```python
from build123d import *

# Parameters (mm, degrees)
EXTRUDE_1_DEPTH     = 20
SKETCH_3_R          = 2.5
CUT_EXTRUDE_1_DEPTH = 4
SKETCH_4_R          = 1.5
CUT_EXTRUDE_2_DEPTH = 14
SKETCH_5_W          = 7.5
SKETCH_5_H          = 8
EXTRUDE_2_DEPTH     = 30
SKETCH_6_R          = 3
CUT_EXTRUDE_3_DEPTH = 6
SKETCH_7_R          = 1.5
CUT_EXTRUDE_4_DEPTH = 6
CHAMFER_1_SIZE      = 2
FILLET_1_R          = 2


with BuildPart() as part:
    # 草图1 → 凸台-拉伸1 (new body)
    with BuildSketch(Plane(origin=(0, 0, 0), x_dir=(1, 0, 0), z_dir=(0, 1, 0))):
        with BuildLine():
            Line((-10.8, 0), (-0.8, 0))
            ThreePointArc((-0.8, 0), (0, 0.8), (0.8, 0))
            Line((0.8, 0), (2.2, 0))
            ThreePointArc((2.2, 0), (3, 0.8), (3.8, 0))
            Line((3.8, 0), (5.2, 0))
            ThreePointArc((5.2, 0), (6, 0.8), (6.8, 0))
            Line((6.8, 0), (8.2, 0))
            ThreePointArc((8.2, 0), (9, 0.8), (9.8, 0))
            Line((9.8, 0), (11.2, 0))
            ThreePointArc((11.2, 0), (12, 0.8), (12.8, 0))
            Line((12.8, 0), (14.2, 0))
            ThreePointArc((14.2, 0), (15, 0.8), (15.8, 0))
            Line((15.8, 0), (17.2, 0))
            ThreePointArc((17.2, 0), (18, 0.8), (18.8, 0))
            Line((18.8, 0), (20.2, 0))
            ThreePointArc((20.2, 0), (21, 0.8), (21.8, 0))
            Line((21.8, 0), (23.2, 0))
            ThreePointArc((23.2, 0), (24, 0.8), (24.8, 0))
            Line((24.8, 0), (26.2, 0))
            ThreePointArc((26.2, 0), (27, 0.8), (27.8, 0))
            Line((27.8, 0), (29.2, 0))
            ThreePointArc((29.2, 0), (30, 0.8), (30.8, 0))
            Line((30.8, 0), (32.2, 0))
            ThreePointArc((32.2, 0), (33, 0.8), (33.8, 0))
            Line((33.8, 0), (35.2, 0))
            ThreePointArc((35.2, 0), (36, 0.8), (36.8, 0))
            Line((36.8, 0), (38.2, 0))
            ThreePointArc((38.2, 0), (39, 0.8), (39.8, 0))
            Line((39.8, 0), (41.2, 0))
            ThreePointArc((41.2, 0), (42, 0.8), (42.8, 0))
            Line((42.8, 0), (44.2, 0))
            ThreePointArc((44.2, 0), (45, 0.8), (45.8, 0))
            Line((45.8, 0), (55.8, 0))
            Line((55.8, 0), (55.8, 8))
            Line((55.8, 8), (-10.8, 8))
            Line((-10.8, 8), (-10.8, 0))
        make_face()
    extrude(amount=EXTRUDE_1_DEPTH)

    # 草图3 → 切除-拉伸1 (cut)
    with BuildSketch(Plane.XY):
        with Locations((50.8, 10)):
            Circle(SKETCH_3_R)
        with Locations((-5.8, 10)):
            Circle(SKETCH_3_R)
    extrude(amount=-CUT_EXTRUDE_1_DEPTH, mode=Mode.SUBTRACT)

    # 草图4 → 切除-拉伸2 (cut)
    with BuildSketch(Plane.XY.offset(-4)):
        with Locations((-5.8, 10)):
            Circle(SKETCH_4_R)
        with Locations((50.8, 10)):
            Circle(SKETCH_4_R)
    extrude(amount=-CUT_EXTRUDE_2_DEPTH, mode=Mode.SUBTRACT)

    # 草图5 → 凸台-拉伸2 (add)
    with BuildSketch(Plane(origin=(0, 20, 0), x_dir=(1, 0, 0), z_dir=(0, 1, 0))):
        with Locations((-7.05, 4)):
            Rectangle(SKETCH_5_W, SKETCH_5_H)
        with Locations((52.05, 4)):
            Rectangle(SKETCH_5_W, SKETCH_5_H)
    extrude(amount=EXTRUDE_2_DEPTH)

    # 草图6 → 切除-拉伸3 (cut)
    with BuildSketch(Plane.XY):
        with Locations((-7.05, 40)):
            Circle(SKETCH_6_R)
        with Locations((52.05, 40)):
            Circle(SKETCH_6_R)
    extrude(amount=-CUT_EXTRUDE_3_DEPTH, mode=Mode.SUBTRACT)

    # 草图7 → 切除-拉伸4 (cut)
    with BuildSketch(Plane.XY.offset(-6)):
        with Locations((-7.05, 40)):
            Circle(SKETCH_7_R)
        with Locations((52.05, 40)):
            Circle(SKETCH_7_R)
    extrude(amount=-CUT_EXTRUDE_4_DEPTH, mode=Mode.SUBTRACT)

    # 倒角1
    chamfer_1_edges = [part.edges().sort_by_distance(p)[0] for p in [
        (-3.3, 20, -4),
        (48.3, 20, -4),
    ]]
    chamfer(chamfer_1_edges, length=CHAMFER_1_SIZE)

    # 圆角1
    fillet_1_edges = [part.edges().sort_by_distance(p)[0] for p in [
        (-10.8, 50, -4),
        (-3.3, 50, -4),
        (55.8, 50, -4),
        (48.3, 50, -4),
    ]]
    fillet(fillet_1_edges, radius=FILLET_1_R)


solid = part.part
```
Build history of the part. All positions in model axes, mm. A direction names the side the tool comes from. Round coordinates to 2 decimals unless told otherwise and drop trailing zeros. Write each loop counter-clockwise with the first axis right and the second up, starting at its lowest first coordinate (ties: lowest second). Pieces come first, ordered by that corner, then holes. Notation, with made-up numbers: (-21.75, 65.25) - (29.25, 65.25) arc R22 cw to (29.25, 86.25) - close; hole circle Ø4 at (58.25, 79.25). An arc over 180 degrees is marked (long way). Write each question's results on one line, items separated by ' | '. Start each with the question number.
Item 1: Which spindle directions (+Z, -Z, +X, -X, +Y, -Y) get a long thin tool onto all of the face, cutting with end or side? Do faces 1 (the face through (45, 9.9, -0.8)), 2 (the face through (-3.87, 49.4, -4.06)), 3 (the face through (-6, 8, -4)). Say none if no direction does.
Item 2: Saw through at A-A (y = 40). Write the cut outline in (x, z), and give its area (3 significant figures).
Item 3: Saw through at B-B (z = -1.5). Write the cut outline in (x, y), and give its area (3 significant figures).
Item 4: Saw through at C-C (y = 34). Write the cut outline in (x, z), and give its area (3 significant figures).
Item 5: Wall check: L1, parallel to X at y = 43.5, z = -4; L2, parallel to X at y = 11, z = -1; L3, parallel to Y at x = 50.8, z = -2.4. Give the ranges that are in metal, low to high. Write a range as [from, to].
Item 6: Drop flat-ended pins along their axis: P1, Ø4, axis at x = -5.8, y = 10, coming from the +Z side; P2, Ø1, axis at x = 15.5, z = -2.5, coming from the -Y side; P3, Ø4, axis at x = 13.5, z = -4.5, coming from the +Y side; P4, Ø5, axis at x = 52.05, y = 40, coming from the +Z side. Give the stop position or say it passes through.
Item 7: Mould opens along Y. For faces 4 (the face through (52.74, 38.67, -6.99)), 5 (the face through (-2.3, 21, -3.9)), 6 (the face through (-7, 43, -3)), 7 (the face through (13, 10, 0)) say: pulls with the +Y half, pulls with the -Y half, needs draft (parallel to the pull), parting line crosses it, or undercut.
Item 8: Saw through at D-D (x = 30). Write the cut outline in (y, z).
Results are:
1) face 1: +Z, +Y, -Y | face 2: +Z, -Z, +Y | face 3: +Z
2) outline: (-10.8, -8) - (-8.55, -8) - (-8.55, -6) - (-10.05, -6) - (-10.05, 0) - (-10.8, 0) - close; (-5.55, -8) - (-3.3, -8) - (-3.3, 0) - (-4.05, 0) - (-4.05, -6) - (-5.55, -6) - close; (48.3, -8) - (50.55, -8) - (50.55, -6) - (49.05, -6) - (49.05, 0) - (48.3, 0) - close; (53.55, -8) - (55.8, -8) - (55.8, 0) - (55.05, 0) - (55.05, -6) - (53.55, -6) - close | area: 36.0 mm²
3) outline: (-10.8, 0) - (55.8, 0) - (55.8, 48) arc R2 ccw to (53.8, 50) - (50.3, 50) arc R2 ccw to (48.3, 48) - (48.3, 22) - (46.3, 20) - (-1.3, 20) - (-3.3, 22) - (-3.3, 48) arc R2 ccw to (-5.3, 50) - (-8.8, 50) arc R2 ccw to (-10.8, 48) - close; hole circle Ø6 at (-7.05, 40); hole circle Ø5 at (-5.8, 10); hole circle Ø5 at (50.8, 10); hole circle Ø6 at (52.05, 40) | area: 1,690 mm²
4) outline: (-10.8, -8) - (-3.3, -8) - (-3.3, 0) - (-10.8, 0) - close; (48.3, -8) - (55.8, -8) - (55.8, 0) - (48.3, 0) - close | area: 120 mm²
5) L1: x = [-10.8, -3.3], [48.3, 55.8] | L2: x = [-10.8, -8.09], [-3.51, 48.51], [53.09, 55.8] | L3: y = [0, 7.5], [12.5, 37.27], [42.73, 50]
6) P1: stops at z = -4 | P2: stops at y = 0 | P3: stops at y = 20 | P4: stops at z = -6
7) face 4: undercut | face 5: pulls with the +Y half | face 6: undercut | face 7: needs draft
8) outline: (0, -8) - (20, -8) - (20, -0.8) - (0, -0.8) - close
